Here's how the part is built. I have some questions about the finished solid (model axes, mm). A direction names the side the tool comes from. Round coordinates to 2 decimals unless told otherwise and drop trailing zeros. Write each loop counter-clockwise with the first axis right and the second up, starting at its lowest first coordinate (ties: lowest second). Pieces come first, ordered by that corner, then holes. Notation, with made-up numbers: (17.25, 72) - (66.25, 72) arc R12 ccw to (66.25, 82) - close; hole circle Ø3 at (0, -24). An arc over 180 degrees is marked (long way). Write item = value, one per line. Start each with the question number.
Item 1: Thinking about a two-plate mould opening in Z: for faces 6 (the face through (3.7, 1.52, 0.08)), 7 (the face through (3, 0, 8)), 8 (the face through (3.69, -1.54, 0.08)), 9 (the face through (3, 0, -8)), which applies, pulls with the +Z half, pulls with the -Z half, needs draft (parallel to the pull), parting line crosses it, or undercut?
Item 2: Which directions (+Z, -Z, +X, -X, +Y, -Y) give clear straight access to the entire face, cutting with the end or side of a thin tool? Please do faces 1 (the face through (2.613, 3.695, 0.084)), 2 (the face through (3.686, 2.6, 0.084)), 3 (the face through (3.53, -3.54, 0.08)), 4 (the face through (0, -5, 0)), 5 (the face through (1, -5, -6)).
Item 3: If we section it at A-A (x = 0): Please give me the cut outline in (y, z), and give its area (3 significant figures).
Item 4: For P1, Ø0.7, axis at x = 0, z = -2.5, coming from the +Y side; P2, Ø1.1, axis at y = 0, z = 1.5, coming from the +X side; P3, Ø1.5, axis at x = -0.5, z = 1.5, coming from the -Y side, each with a flat end and sliding along its axis, tell me the tip position at first contact or that it passes through.
Item 5: If I drill on line 1 along Y through (x, z) = (0, -4); line 2 along Y through (x, z) = (3.5, 5.5), over which ranges is the centre line in solid material (lowest first)? Write a range as [from, to].
```python
from build123d import *

# Parameters (mm, degrees)
SKETCH1_R               = 4
BOSS_EXTRUDE1_DEPTH     = 6
SKETCH2_R               = 7
BOSS_EXTRUDE2_DEPTH     = 2
LPATTERN1_COUNT         = 2
LPATTERN1_PITCH         = 14
CUT_EXTRUDE1_DEPTH      = 13.727922061
CUT_EXTRUDE1_DEPTH_BACK = 13.727922061
SKETCH3_R               = 2.5
CHAMFER1_SIZE           = 1
BOSS_EXTRUDE3_DEPTH     = 6
CIRPATTERN1_COUNT       = 8


with BuildPart() as part:
    # Sketch1 → Boss-Extrude1 (new, symmetric)
    with BuildSketch(Plane.XY):
        Circle(SKETCH1_R)
    extrude(amount=BOSS_EXTRUDE1_DEPTH, both=True)

    # Sketch2 → Boss-Extrude2 (add)
    with BuildSketch(Plane.XY.offset(6)):
        Circle(SKETCH2_R)
    boss_extrude2 = extrude(amount=BOSS_EXTRUDE2_DEPTH)

    # LPattern1: Boss-Extrude2 ×2
    with Locations(*[(0, 0, -i * LPATTERN1_PITCH) for i in range(1, LPATTERN1_COUNT)]):
        add(boss_extrude2)

    # Sketch3 → Cut-Extrude1 (cut, two sides: drawn at the far end of the back side and taken through both)
    with BuildSketch(Plane.XY.offset(-CUT_EXTRUDE1_DEPTH_BACK)):
        Circle(SKETCH3_R)
    extrude(amount=CUT_EXTRUDE1_DEPTH + CUT_EXTRUDE1_DEPTH_BACK, mode=Mode.SUBTRACT)

    # Chamfer1
    chamfer1_edges = [part.edges().sort_by_distance(p)[0] for p in [
        (-7, 0, 8),
        (-7, 0, -8),
    ]]
    chamfer(chamfer1_edges, length=CHAMFER1_SIZE)

    # Sketch6 → Boss-Extrude3 (add, symmetric)
    with BuildSketch(Plane.XY):
        Polygon((1.1, 2.6), (0.668195185, 5), (-0.668195185, 5), (-1.1, 2.6), align=None)
    boss_extrude3 = extrude(amount=BOSS_EXTRUDE3_DEPTH, both=True)

    # CirPattern1: Boss-Extrude3 ×8 about axis
    cirpattern1_axis = Axis((0, 0, 0), (0, 0, 1))
    for i in range(1, CIRPATTERN1_COUNT):
        add(boss_extrude3.rotate(cirpattern1_axis, i * 360 / CIRPATTERN1_COUNT))


solid = part.part
```
Reply:
q1.face_6 = undercut
q1.face_7 = pulls with the +Z half
q1.face_8 = undercut
q1.face_9 = pulls with the -Z half
q2.face_1 = +Y
q2.face_2 = +X
q2.face_3 = +X, -Y
q2.face_4 = +X, -X, -Y
q2.face_5 = none
q3.outline = (-7, -7) - (-6, -8) - (-2.5, -8) - (-2.5, 8) - (-6, 8) - (-7, 7) - (-7, 6) - (-5, 6) - (-5, -6) - (-7, -6) - close; (2.5, -8) - (6, -8) - (7, -7) - (7, -6) - (5, -6) - (5, 6) - (7, 6) - (7, 7) - (6, 8) - (2.5, 8) - close
q3.area = 94.0 mm2
q4.P1 = 5
q4.P2 = 5
q4.P3 = -5
q5.line_1 = [-5, -2.5], [2.5, 5]
q5.line_2 = [-3.57, -2.33], [-1.94, 1.94], [2.33, 3.57]
